```python
from build123d import *

# Parameters (mm, degrees)
F0_R     = 2.5
F1_DEPTH = 14
F2_W     = 12.5
F2_H     = 16.927838
F3_DEPTH = 20
F5_DEPTH = 5.85
F6_W     = 9.7
F6_H     = 13.5
F7_DEPTH = 26.2
F8_R     = 2


with BuildPart() as f1:
    # F0 (on Front) → F1 (new body)
    with BuildSketch(Plane.XZ):
        with BuildLine():
            Line((7.5, 0), (7.5, 8.2))
            ThreePointArc((7.5, 8.2), (0, 15.7), (-7.5, 8.2))
            Line((-7.5, 8.2), (-7.5, 0))
            Line((-7.5, 0), (7.5, 0))
        make_face()
        with Locations((0, 8.2)):
            Circle(F0_R, mode=Mode.SUBTRACT)
    extrude(amount=F1_DEPTH)

    # F2 (on Right) → F3 (cut, symmetric)
    with BuildSketch(Plane.YZ):
        with Locations((-7.75, 9.963919)):
            Rectangle(F2_W, F2_H)
    extrude(amount=F3_DEPTH, both=True, mode=Mode.SUBTRACT)

    # F4 (on Right) → F5 (join, symmetric)
    with BuildSketch(Plane.YZ):
        Polygon((-1.5, 1.5), (-1.5, 10.4), (-10.4, 1.5), align=None)
    extrude(amount=F5_DEPTH, both=True)

    # F6 (on face) → F7 (cut)
    with BuildSketch(Plane.XY.offset(1.5)):
        with Locations((0, -8.25)):
            Rectangle(F6_W, F6_H)
    extrude(amount=F7_DEPTH, mode=Mode.SUBTRACT)

    # F8
    f8_edges = [f1.edges().sort_by_distance(p)[0] for p in [
        (7.5, -14, 0.75),
        (-7.5, -14, 0.75),
    ]]
    fillet(f8_edges, radius=F8_R)


solid = f1.part
```
Work out the finished part from the listing and answer in its coordinate system (mm). A direction names the side the tool comes from. Coordinates: 2 decimals unless noted, no trailing zeros. Order: outer loops, then holes, each group sorted by start corner. A loop starts at its lowest first (then second) coordinate and runs counter-clockwise, first axis right, second up. Notation, with made-up numbers: (-4.75, 45.25) - (9.25, 45.25) arc R11 cw to (9.25, 63.25) - close; hole circle Ø5 at (53, -37). An arc over 180 degrees is marked (long way). Answer as a JSON object with one key per item and string values.
1. Find section A-A on x = 0. Determine the outline of the cut face in (y, z), plus the area to 3 significant figures.
Output values:
{"outline": "(-14, 0) - (0, 0) - (0, 5.7) - (-1.5, 5.7) - (-1.5, 1.5) - (-14, 1.5) - close; (-1.5, 10.7) - (0, 10.7) - (0, 15.7) - (-1.5, 15.7) - close", "area": "34.8 mm²"}
2. A tool of negligible diameter and unlimited length cuts with its end or side. For faces 1 (the face through (-4.85, -4, 4)), 2 (the face through (-5.85, -4, 4)), 3 (the face through (5.85, -4, 4)), from which of +Z, -Z, +X, -X, +Y, -Y can it reach the whole face along a straight path? Write none if from no direction.
Output values:
{"face 1": "+Z, -Y", "face 2": "+Z, -X, -Y", "face 3": "+Z, +X, -Y"}
3. Find section D-D on y = -6.25. Determine the outline of the cut face in (x, z).
Output values:
{"outline": "(-7.5, 0) - (7.5, 0) - (7.5, 1.5) - (5.85, 1.5) - (5.85, 5.65) - (4.85, 5.65) - (4.85, 1.5) - (-4.85, 1.5) - (-4.85, 5.65) - (-5.85, 5.65) - (-5.85, 1.5) - (-7.5, 1.5) - close"}
4. Find section B-B on z = 7.25. Determine the outline of the cut face in (x, y), plus the area to 3 significant figures.
Output values:
{"outline": "(-7.5, -1.5) - (-5.85, -1.5) - (-5.85, -4.65) - (-4.85, -4.65) - (-4.85, -1.5) - (-2.31, -1.5) - (-2.31, 0) - (-7.5, 0) - close; (2.31, -1.5) - (4.85, -1.5) - (4.85, -4.65) - (5.85, -4.65) - (5.85, -1.5) - (7.5, -1.5) - (7.5, 0) - (2.31, 0) - close", "area": "21.9 mm²"}
5. Each of these flat-tipped pins is pushed along its axis until it touches: P1, Ø7, axis at y = -7.5, z = 4.5, coming from the +X side; P2, Ø1.5, axis at x = 5, y = -2.5, coming from the +Z side; P3, Ø1, axis at x = -2, y = -8, coming from the +Z side; P4, Ø2, axis at x = -5, y = -5, coming from the +Z side. Where does it stop, or does it pass through?
Output values:
{"P1": "stops at x = 7.5", "P2": "stops at z = 10.15", "P3": "stops at z = 1.5", "P4": "stops at z = 7.9"}
6. The mould has two halves that part along X. Classify faces 4 (the face through (-6.9, -13.43, 0.74)), 5 (the face through (0, -8, 1.5)), 6 (the face through (-5.3, -5.9, 6)): +X half, -X half, draft (parallel to the pull), parting line (faces both ways), or undercut.
Output values:
{"face 4": "-X half", "face 5": "undercut", "face 6": "draft"}
7. Consider line 1 (X direction, y = -3.75, z = 6.75); line 2 (Z direction, x = 0, y = -1.2); line 3 (Y direction, x = -4, z = 10.25). Determine where each line is inside the solid, lowest interval first.
Output values:
{"line 1": "x = -5.85 to -4.85, 4.85 to 5.85", "line 2": "z = 0 to 5.7, 10.7 to 15.7", "line 3": "y = -1.5 to 0"}
8. Find section C-C on z = 5. Determine the outline of the cut face in (x, y).
Output values:
{"outline": "(-7.5, -1.5) - (-5.85, -1.5) - (-5.85, -6.9) - (-4.85, -6.9) - (-4.85, -1.5) - (4.85, -1.5) - (4.85, -6.9) - (5.85, -6.9) - (5.85, -1.5) - (7.5, -1.5) - (7.5, 0) - (-7.5, 0) - close"}
